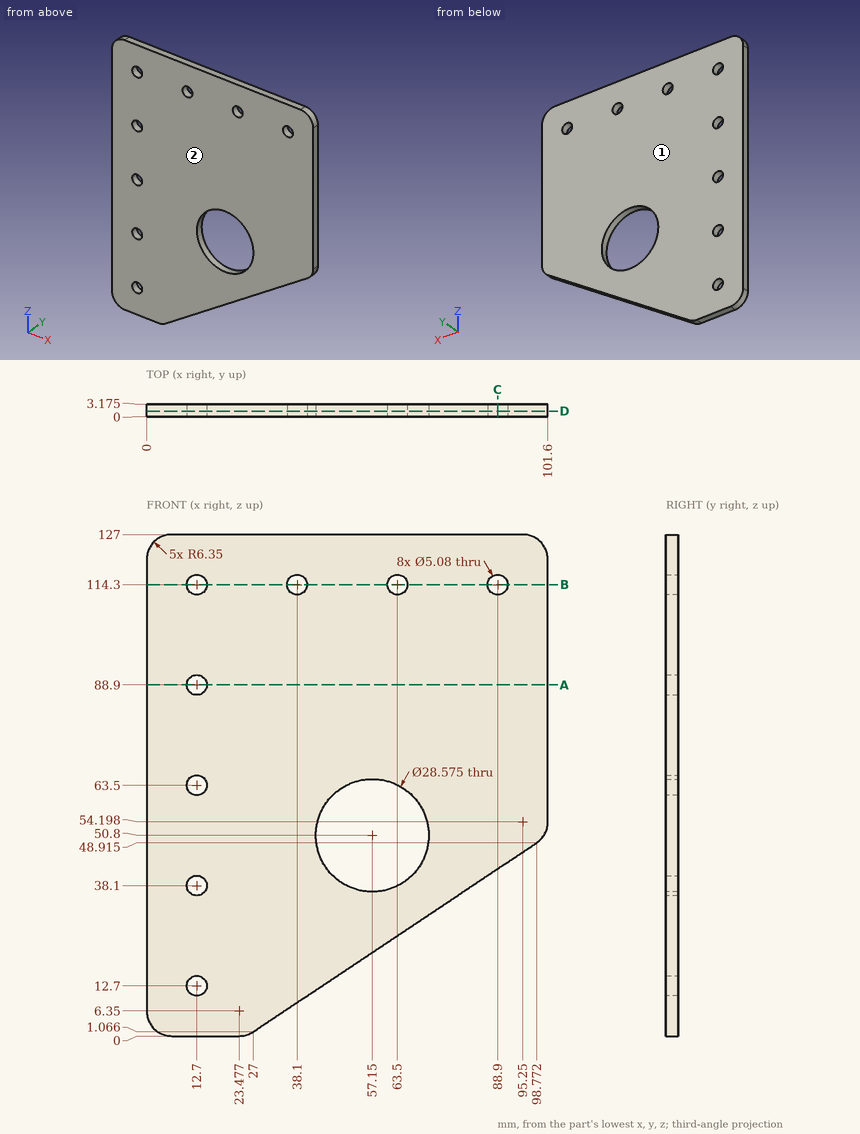
Can you work these out from the drawing? Everything is in mm from the part's minimum corner. Give positions to 0.01 mm unless a question says otherwise; leave off trailing zeros. Loops run counter-clockwise (first coordinate to the right, second up) from the corner with the lowest first, then second, coordinate; pieces in that order, holes last. Notation, with made-up numbers: (87, 36.5) -> (133, 36.5) arc R31 ccw to (133, 70.5) -> close; hole circle Ø3 at (12.5, 63.5). An arc over 180 degrees is marked (long way). Return JSON: item names as keys, results as strings.
Item 1: We'd pull the mould along Y, two halves only. Please class the marked faces 1 and 2: +Y half, -Y half, draft (parallel to the pull), parting line (faces both ways), or undercut.
Geometry results:
{"face 1": "+Y half", "face 2": "-Y half"}
Item 2: If we section it at D-D on y = 1.4: Count the separate pieces of the cut face and the enclosed holes in it, plus the area to 3 significant figures.
Geometry results:
{"separate pieces": "1", "enclosed holes": "9", "area": "10,100 mm²"}
Item 3: If we section it at C-C on x = 88.9: List the corners of the cut face in (y, z) for me (1 decimal), plus the area to 3 significant figures.
Geometry results:
{"outline": "(0, 42.3) -> (3.2, 42.3) -> (3.2, 111.8) -> (0, 111.8) -> close; (0, 116.8) -> (3.2, 116.8) -> (3.2, 127) -> (0, 127) -> close", "area": "253 mm²"}
Item 4: If we section it at B-B on z = 114.3: List the corners of the cut face in (x, y) for me (1 decimal), plus the area to 3 significant figures.
Geometry results:
{"outline": "(0, 0) -> (10.2, 0) -> (10.2, 3.2) -> (0, 3.2) -> close; (15.2, 0) -> (35.6, 0) -> (35.6, 3.2) -> (15.2, 3.2) -> close; (40.6, 0) -> (61, 0) -> (61, 3.2) -> (40.6, 3.2) -> close; (66, 0) -> (86.4, 0) -> (86.4, 3.2) -> (66, 3.2) -> close; (91.4, 0) -> (101.6, 0) -> (101.6, 3.2) -> (91.4, 3.2) -> close", "area": "258 mm²"}
Item 5: If we section it at A-A on z = 88.9: List the corners of the cut face in (x, y) for me (1 decimal).
Geometry results:
{"outline": "(0, 0) -> (10.2, 0) -> (10.2, 3.2) -> (0, 3.2) -> close; (15.2, 0) -> (101.6, 0) -> (101.6, 3.2) -> (15.2, 3.2) -> close"}
Item 6: I'm going to push flat-ended pins straight in: pin 1 (4 mm diameter, centred on x = 12.7, z = 12.7, fed in from +Y); pin 2 (1 mm diameter, centred on x = 37.5, y = 1.5, fed in from -Z); pin 3 (1 mm diameter, centred on y = 0.5, z = 53.5, fed in from +X). Where does each tip first touch, or does it pass through?
Geometry results:
{"pin 1": "passes through", "pin 2": "stops at z = 7.73", "pin 3": "stops at x = 101.6"}
Item 7: I need wall thicknesses on L1, parallel to X at y = 2.3, z = 114.3; L2, parallel to X at y = 1, z = 88.9; L3, parallel to X at y = 1.3, z = 63.5 (1 decimal). Which ranges of each line are inside material? Lowest first, please. Write a range as from..to.
Geometry results:
{"L1": "x = 0..10.16, 15.24..35.56, 40.64..60.96, 66.04..86.36, 91.44..101.6", "L2": "x = 0..10.16, 15.24..101.6", "L3": "x = 0..10.2, 15.2..50.6, 63.7..101.6"}
